Model file for the job. Use its own axes, mm. A direction names the side the tool comes from. Give positions to 0.01 mm unless a question says otherwise; leave off trailing zeros. Loops run counter-clockwise (first coordinate to the right, second up) from the corner with the lowest first, then second, coordinate; pieces in that order, holes last. Notation, with made-up numbers: (-18.5, 80.5) -> (-10.5, 80.5) arc R19 ccw to (-10.5, 86.5) -> close; hole circle Ø1 at (66.5, 86.25). An arc over 180 degrees is marked (long way). Use CSV: the item, a comma, the result in double quotes. Start each with the question number.
(1) Drill centre lines: probe 1 along Y at (x, z) = (-11.75, -0.2); probe 2 along Y at (x, z) = (-8.75, -0.25); probe 3 along Y at (x, z) = (-9.5, -1.8). Where is each one in solid material? Low to high.
(2) Cut at B-B on y = 0. Write the cut outline in (x, z), then the cut area to 3 significant figures.
(3) Cut at C-C on z = -1.3. Write the cut outline in (x, y), then the cut area to 3 significant figures.
(4) Cut at A-A on x = -9.5. Write the cut outline in (y, z), then the cut area to 3 significant figures.
(5) 3-axis set-ups, long thin cutter, end or side, ignore diameter. For faces 1 (the flat face through (-10.83, 4.4, -1.04)), 2 (the flat face through (-8.063, 2.519, -1.035)): which of +Z, -Z, +X, -X, +Y, -Y reach the whole face in a straight line?
(6) Pull direction Y, two halves, no side cores. Call faces 3 (the flat face through (-8, 0, 0)), 4 (the flat face through (-12.51, 5.19, -1.04)), 5 (the flat face through (-12.645, 3.348, -1.035)): pulls with the +Y half, pulls with the -Y half, needs draft (parallel to the pull), parting line crosses it, or undercut.
(7) Cut at D-D on z = -2.65. Write the cut outline in (x, y).
(8) Flat gauge pins, fed straight in: pin 1 (0.6 mm diameter, centred on x = -13.5, z = -1.5, fed in from -Y); pin 2 (0.6 mm diameter, centred on y = -0.5, z = -1, fed in from +X); pin 3 (1.7 mm diameter, centred on x = -5, z = -1, fed in from +Y). Where does each tip first touch, or does it go through?
from build123d import *

# Parameters (mm, degrees)
SKETCH1_R           = 7
SKETCH1_R_2         = 1
BOSS_EXTRUDE1_DEPTH = 3
SKETCH2_W           = 3.1
SKETCH2_H           = 2.1
CUT_EXTRUDE1_DEPTH  = 2.1
CIRPATTERN1_COUNT   = 6
BOSS_EXTRUDE2_DEPTH = 0.4
CIRPATTERN2_COUNT   = 6


with BuildPart() as part:
    # Sketch1 → Boss-Extrude1 (new body)
    with BuildSketch(Plane.XY):
        with Locations((-9.5, 0)):
            Circle(SKETCH1_R)
        with Locations((-9.5, 0)):
            Circle(SKETCH1_R_2, mode=Mode.SUBTRACT)
    extrude(amount=-BOSS_EXTRUDE1_DEPTH)

    # Sketch2 → Cut-Extrude1 (cut)
    with BuildSketch(Plane.XY):
        with Locations((-13.95, 0)):
            Rectangle(SKETCH2_W, SKETCH2_H)
    cut_extrude1 = extrude(amount=-CUT_EXTRUDE1_DEPTH, mode=Mode.SUBTRACT)

    # CirPattern1: Cut-Extrude1 ×6 about axis
    cirpattern1_axis = Axis((-9.5, 0, 0), (0, 0, 1))
    for i in range(1, CIRPATTERN1_COUNT):
        add(cut_extrude1.rotate(cirpattern1_axis, i * 360 / CIRPATTERN1_COUNT), mode=Mode.SUBTRACT)

    # Sketch3 → Boss-Extrude2 (add)
    with BuildSketch(Plane.XY):
        with BuildLine():
            Line((-14.5, -1.05), (-13.5, -1.05))
            ThreePointArc((-13.5, -1.05), (-14, -0.8744998), (-14.5, -1.05))
        make_face()
        with BuildLine():
            Line((-14.5, 1.05), (-13.5, 1.05))
            ThreePointArc((-13.5, 1.05), (-14, 0.8744998), (-14.5, 1.05))
        make_face()
    boss_extrude2 = extrude(amount=-BOSS_EXTRUDE2_DEPTH)

    # CirPattern2: Boss-Extrude2 ×6 about axis
    cirpattern2_axis = Axis((-9.5, 0, 0), (0, 0, 1))
    for i in range(1, CIRPATTERN2_COUNT):
        add(boss_extrude2.rotate(cirpattern2_axis, i * 360 / CIRPATTERN2_COUNT))


solid = part.part
Check result:
1,probe 1,"-6.63 to -5.63, -2.05 to 2.05, 5.63 to 6.63"
1,probe 2,"-6.96 to -3.4, -2.92 to -0.66, 0.66 to 2.92, 3.4 to 6.96"
1,probe 3,"-7 to -1, 1 to 7"
2,outline,"(-16.5, -3) -> (-10.5, -3) -> (-10.5, 0) -> (-12.4, 0) -> (-12.4, -2.1) -> (-15.5, -2.1) -> (-15.5, 0) -> (-16.5, 0) -> close; (-8.5, -3) -> (-2.5, -3) -> (-2.5, 0) -> (-3.5, 0) -> (-3.5, -2.1) -> (-6.6, -2.1) -> (-6.6, 0) -> (-8.5, 0) -> close"
2,area,"23.0 mm²"
3,outline,"circle Ø14 at (-9.5, 0); hole (-15.5, -1.05) -> (-12.4, -1.05) -> (-12.4, 1.05) -> (-15.5, 1.05) -> close; hole (-13.41, -4.67) -> (-11.59, -5.72) -> (-10.04, -3.04) -> (-11.86, -1.99) -> close; hole (-13.41, 4.67) -> (-11.86, 1.99) -> (-10.04, 3.04) -> (-11.59, 5.72) -> close; hole circle Ø2 at (-9.5, 0); hole (-8.96, -3.04) -> (-7.41, -5.72) -> (-5.59, -4.67) -> (-7.14, -1.99) -> close; hole (-8.96, 3.04) -> (-7.14, 1.99) -> (-5.59, 4.67) -> (-7.41, 5.72) -> close; hole (-6.6, -1.05) -> (-3.5, -1.05) -> (-3.5, 1.05) -> (-6.6, 1.05) -> close"
3,area,"112 mm²"
4,outline,"(-7, -3) -> (-1, -3) -> (-1, 0) -> (-7, 0) -> close; (1, -3) -> (7, -3) -> (7, 0) -> (1, 0) -> close"
4,area,"36.0 mm²"
5,face 1,"none"
5,face 2,"+Z"
6,face 3,"needs draft"
6,face 4,"undercut"
6,face 5,"undercut"
7,outline,"circle Ø14 at (-9.5, 0); hole circle Ø2 at (-9.5, 0)"
8,pin 1,"y = -5.94"
8,pin 2,"x = -2.5"
8,pin 3,"y = 5.97"
